The model under review builds one solid part; all positions refer to its coordinate system, in mm. Face numbers are marked on the shaded views. A direction names the side the tool comes from. Round coordinates to 2 decimals unless told otherwise and drop trailing zeros. Order: outer loops, then holes, each group sorted by start corner. A loop starts at its lowest first (then second) coordinate and runs counter-clockwise, first axis right, second up. Notation, with made-up numbers: M -9.75,25 L 6.25,25 A20 ccw 6.25,41 Z; hole C -39.5,13 d6. An arc over 180 degrees is marked long. Answer as CSV lines item,"result". Start each with the question number.
from build123d import *

# Parameters (mm, degrees)
SKETCH1_W               = 17
SKETCH1_H               = 15
BOSS_EXTRUDE1_DEPTH     = 5
SKETCH2_W               = 3
SKETCH2_H               = 15
SKETCH2_H_2             = 14.97636143
BOSS_EXTRUDE2_DEPTH     = 5
CUT_EXTRUDE2_DEPTH      = 21.185301583
CUT_EXTRUDE2_DEPTH_BACK = 21.185301583
SKETCH4_R               = 1.5
FILLET1_R               = 6
FILLET3_RADIUS          = 1.5
FILLET3_LENGTH          = 14.97636143
FILLET4_RADIUS          = 1.5
FILLET4_LENGTH          = 15
SKETCH5_W               = 1.007967197
SKETCH5_H               = 15
SKETCH5_W_2             = 1.056413299
CUT_EXTRUDE4_DEPTH      = 10


with BuildPart() as part:
    # Sketch1 → Boss-Extrude1 (new body)
    with BuildSketch(Plane.XY):
        with Locations((-8.5, -7.5)):
            Rectangle(SKETCH1_W, SKETCH1_H)
    extrude(amount=BOSS_EXTRUDE1_DEPTH)

    # Sketch2 → Boss-Extrude2 (add)
    with BuildSketch(Plane.XY.offset(5)):
        with Locations((-6.42, -7.5)):
            Rectangle(SKETCH2_W, SKETCH2_H)
        with Locations((-10.58, -7.511819285)):
            Rectangle(SKETCH2_W, SKETCH2_H_2)
    extrude(amount=BOSS_EXTRUDE2_DEPTH)

    # Sketch4 → Cut-Extrude2 (cut, two sides: drawn at the far end of the back side and taken through both)
    with BuildSketch(Plane(origin=(-9.08, 0, 0), x_dir=(0, 0, -1), z_dir=(1, 0, 0)).offset(-CUT_EXTRUDE2_DEPTH_BACK)):
        with Locations(Location((-7.041389116, -7.762480296, 0), (0, 0, 270))):
            Circle(SKETCH4_R)
    extrude(amount=CUT_EXTRUDE2_DEPTH + CUT_EXTRUDE2_DEPTH_BACK, mode=Mode.SUBTRACT)

    # Fillet1
    # the kernel refuses this fillet: 6 mm, written as the material it takes off along each edge
    with BuildSketch(Plane(origin=(0, -29.754999153, 5), x_dir=(0, 0, -1), z_dir=(0, 1, 0))) as fillet1_piece_1:
        with BuildLine():
            CenterArc((5.901999661, 6), FILLET1_R, 190.369759805, 79.630240195)
            Line((0, 4.92), (0, 0))
            Line((0, 0), (5.901999661, 0))
        make_face()
    extrude(amount=44.509998306, mode=Mode.SUBTRACT)
    # the kernel refuses this fillet: 6 mm, written as the material it takes off along each edge
    with BuildSketch(Plane(origin=(-17, 14.790199458, 5), x_dir=(0, 0, -1), z_dir=(0, -1, 0))) as fillet1_2_piece_1_section:
        with BuildLine():
            CenterArc((6, 5.916079783), FILLET1_R, 180, 80.405931773)
            Line((0, 5.916079783), (0, 0))
            Line((0, 0), (5, 0))
        make_face()
    fillet1_2_piece_1 = extrude(amount=44.580398916, mode=Mode.PRIVATE)
    fillet1_2_piece_1 = split(fillet1_2_piece_1, bisect_by=Plane(origin=(-17, -0.02363857, 5), z_dir=(0, 1, 0)), keep=Keep.TOP, mode=Mode.PRIVATE)
    fillet1_2_piece_1 = split(fillet1_2_piece_1, bisect_by=Plane(origin=(-12.08, 14.790199458, 5), z_dir=(-1, 0, 0)), keep=Keep.TOP, mode=Mode.PRIVATE)
    add(fillet1_2_piece_1, mode=Mode.SUBTRACT)
    with BuildSketch(Plane(origin=(-17, 14.790199458, 5), x_dir=(0, 0, -1), z_dir=(0, -1, 0))) as fillet1_2_piece_2_section:
        with BuildLine():
            CenterArc((6, 5.916079783), FILLET1_R, 180, 80.405931773)
            Line((0, 5.916079783), (0, 0))
            Line((0, 0), (5, 0))
        make_face()
    fillet1_2_piece_2 = extrude(amount=44.580398916, mode=Mode.PRIVATE)
    fillet1_2_piece_2 = split(fillet1_2_piece_2, bisect_by=Plane(origin=(-17, -0.02363857, 5), z_dir=(0, 1, 0)), keep=Keep.TOP, mode=Mode.PRIVATE)
    fillet1_2_piece_2 = split(fillet1_2_piece_2, bisect_by=Plane(origin=(-12.08, 14.790199458, 5), z_dir=(1, 0, 0)), keep=Keep.TOP, mode=Mode.PRIVATE)
    add(fillet1_2_piece_2, mode=Mode.SUBTRACT)
    with BuildSketch(Plane(origin=(-17, 14.790199458, 5), x_dir=(0, 0, -1), z_dir=(0, -1, 0))) as fillet1_2_piece_3_section:
        with BuildLine():
            CenterArc((6, 5.916079783), FILLET1_R, 180, 80.405931773)
            Line((0, 5.916079783), (0, 0))
            Line((0, 0), (5, 0))
        make_face()
    fillet1_2_piece_3 = extrude(amount=44.580398916, mode=Mode.PRIVATE)
    fillet1_2_piece_3 = split(fillet1_2_piece_3, bisect_by=Plane(origin=(-17, -0.02363857, 5), z_dir=(0, -1, 0)), keep=Keep.TOP, mode=Mode.PRIVATE)
    fillet1_2_piece_3 = split(fillet1_2_piece_3, bisect_by=Plane(origin=(-12.08, 14.790199458, 5), z_dir=(-1, 0, 0)), keep=Keep.TOP, mode=Mode.PRIVATE)
    add(fillet1_2_piece_3, mode=Mode.SUBTRACT)

    # Fillet3: full round fillet: the end face becomes a half cylinder, R = half its width
    fillet3_face = Plane((-10.58, -7.511819285, 10), x_dir=(0, -1, 0), z_dir=(0, 0, 1))  # on the end face: x along it, z out of the body
    fillet3_slab = fillet3_face.offset(-FILLET3_RADIUS / 2) * Box(FILLET3_LENGTH, 2 * FILLET3_RADIUS, FILLET3_RADIUS, mode=Mode.PRIVATE)  # the body's end, R deep
    fillet3_round = Plane((-10.58, -7.511819285, 8.5), x_dir=(0, 0, 1), z_dir=(0, -1, 0)) * Cylinder(FILLET3_RADIUS, FILLET3_LENGTH, mode=Mode.PRIVATE)  # its axis R under the face
    add(fillet3_slab - fillet3_round, mode=Mode.SUBTRACT)

    # Fillet4: full round fillet: the end face becomes a half cylinder, R = half its width
    fillet4_face = Plane((-6.42, -7.5, 10), x_dir=(0, -1, 0), z_dir=(0, 0, 1))  # on the end face: x along it, z out of the body
    fillet4_slab = fillet4_face.offset(-FILLET4_RADIUS / 2) * Box(FILLET4_LENGTH, 2 * FILLET4_RADIUS, FILLET4_RADIUS, mode=Mode.PRIVATE)  # the body's end, R deep
    fillet4_round = Plane((-6.42, -7.5, 8.5), x_dir=(0, 0, 1), z_dir=(0, -1, 0)) * Cylinder(FILLET4_RADIUS, FILLET4_LENGTH, mode=Mode.PRIVATE)  # its axis R under the face
    add(fillet4_slab - fillet4_round, mode=Mode.SUBTRACT)

    # Sketch5 → Cut-Extrude4 (cut)
    with BuildSketch(Plane.XY):
        with Locations((-0.572171345, -7.5)):
            Rectangle(SKETCH5_W, SKETCH5_H)
        with Locations((-16.471793351, -7.5)):
            Rectangle(SKETCH5_W_2, SKETCH5_H)
    extrude(amount=CUT_EXTRUDE4_DEPTH, mode=Mode.SUBTRACT)


solid = part.part
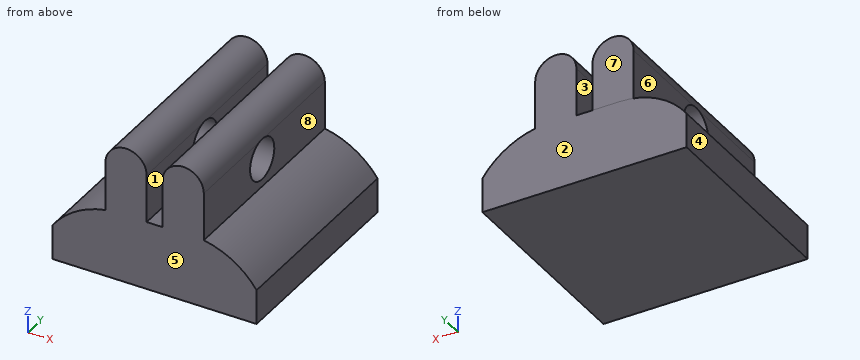
Item 1: For pin 1 (3 mm diameter, centred on y = -9.5, z = 7, fed in from +X); pin 2 (3 mm diameter, centred on y = -6.5, z = 5, fed in from +X); pin 3 (3 mm diameter, centred on y = -5, z = 6.5, fed in from -X), all flat-tipped, find the tip position at first contact; note any pin that passes through.
Item 2: Consider section B-B (z = 7.5). State the section outline as (x, y) points.
Item 3: Wall thickness on probe 1 along X at (y, z) = (-9.25, 8.5); probe 2 along X at (y, z) = (-9, 9.25); probe 3 along Z at (x, y) = (-8.25, -7): over which ranges is each line inside the solid? List them lowest first. Write a range as [from, to].
Item 4: The part is to be moulded in two halves that separate along X. For the marked faces 1, 2, 3 and 4, say which applies: +X half, -X half, draft (parallel to the pull), parting line (faces both ways), or undercut.
Item 5: Tool access review of the marked faces 5, 6, 7 and 8: name each direction out of +Z, -Z, +X, -X, +Y, -Y from which nothing blocks a thin tool from reaching the whole face with its end or side.
Item 6: Consider section A-A (y = -5.5). State the section outline as (x, z) points.
Item 7: Consider section D-D (x = -8.5). State the section outline as (y, z) points, and give its area (3 significant figures).
Reported:
1,pin 1,"stops at x = -4.92"
1,pin 2,"stops at x = -1.92"
1,pin 3,"stops at x = -12.08"
2,outline,"M -12.08,-15 L -9.08,-15 L -9.08,-9.19 L -12.08,-9.19 Z; M -12.08,-6.33 L -9.08,-6.33 L -9.08,-0.02 L -12.08,-0.02 Z; M -7.92,-15 L -4.92,-15 L -4.92,-9.19 L -7.92,-9.19 Z; M -7.92,-6.33 L -4.92,-6.33 L -4.92,0 L -7.92,0 Z"
3,probe 1,"x = [-12.08, -9.08], [-7.92, -4.92]"
3,probe 2,"x = [-11.88, -9.28], [-7.72, -5.12]"
3,probe 3,"z = [0, 5]"
4,face 1,"undercut"
4,face 2,"draft"
4,face 3,"undercut"
4,face 4,"-X half"
5,face 5,"+Z, -Z, +X, -X, -Y"
5,face 6,"+Z, -X, +Y, -Y"
5,face 7,"+Z, -X, +Y"
5,face 8,"+Z, +X, +Y, -Y"
6,outline,"M -15.94,0 L -1.08,0 L -1.08,2.53 A6 ccw -4.92,5 L -4.92,8.5 A1.5 ccw -7.92,8.5 L -7.92,5 L -9.08,5 L -9.08,8.5 A1.5 ccw -12.08,8.5 L -12.08,4.92 A6 ccw -15.94,2.52 Z"
7,outline,"M -15,0 L 0,0 L 0,5 L -15,5 Z"
7,area,"75.0 mm²"
